For this review, take the finished solid that the model builds, in its own axes (mm). Face numbers are marked on the shaded views. A direction names the side the tool comes from. Round coordinates to 2 decimals unless told otherwise and drop trailing zeros. Loops run counter-clockwise (first coordinate to the right, second up) from the corner with the lowest first, then second, coordinate; pieces in that order, holes last. Notation, with made-up numbers: M -11.5,-25 L 14.5,-25 A18 ccw 14.5,-19 Z; hole C 44,75 d7. An arc over 180 degrees is marked long. One line per question, with ' | ' between items. Start each with the question number.
1) We need section D-D (x = 5.25). Give the boundary of the cut face in (y, z), and give its area (3 significant figures).
2) For probe 1 along Z at (x, y) = (-1.5, 46); probe 2 along Y at (x, z) = (4, -2), list the stretches that pass through material, from the lowest coordinate up. Write a range as from..to.
3) We need section B-B (x = 1). Give the boundary of the cut face in (y, z).
4) For pin 1 Ø3 at (x, y) = (2.5, 55) entering from -Z; pin 2 Ø2 at (x, y) = (1, 42.5) entering from +Z; pin 3 Ø6 at (y, z) = (49, 0) entering from +X, all flat-tipped, find the tip position at first contact; note any pin that passes through.
5) We need section A-A (z = -0.5). Give the boundary of the cut face in (x, y), and give its area (3 significant figures).
6) For the marked faces 1, 2, 3, 4 and 5, list the 3-axis set-ups (+Z, -Z, +X, -X, +Y, -Y) from which the entire face can be reached by the end or side of a thin tool; tool diameter is ignored.
7) We need section C-C (y = 16). Give the boundary of the cut face in (x, z), and give its area (3 significant figures).
Autodesk Inventor part; units mm, degrees
ref_plane "YZ Plane" through (0, 0, 0) normal (1, 0, 0) x (0, 1, 0)
ref_plane "XZ Plane" through (0, 0, 0) normal (0, 1, 0) x (-1, 0, 0)
ref_plane "XY Plane" through (0, 0, 0) normal (0, 0, 1) x (1, 0, 0)
sketch "Szkic1" plane through (0, 0, 0) normal (0, 1, 0) x (-1, 0, 0)
  line L0 (-6, 6) -> (6, 6)
  line L1 (6, 6) -> (6, -6)
  line L2 (6, -6) -> (-6, -6)
  line L3 (-6, -6) -> (-6, 6)
  line L4 (-6, 6) -> (6, -6) construction
  line L5 (6, 6) -> (-6, -6) construction
  line L6 (-3.5, 3.5) -> (3.5, 3.5)
  line L7 (3.5, 3.5) -> (3.5, -3.5)
  line L8 (3.5, -3.5) -> (-3.5, -3.5)
  line L9 (-3.5, -3.5) -> (-3.5, 3.5)
  line L10 (-3.5, 3.5) -> (3.5, -3.5) construction
  line L11 (3.5, 3.5) -> (-3.5, -3.5) construction
  point P0 (0, 0)
  dimension "d0" = 12
  dimension "d1" = 12
  dimension "d2" = 7
  dimension "d3" = 7
extrude "Wyciągnięcie proste1" add sketch "Szkic1" along normal blind 72 contours L6 L7 L8 L9
extrude "Wyciągnięcie proste2" add sketch "Szkic1" against normal blind 2 contours L0 L1 L2 L3 | L6 L7 L8 L9
fillet "Zaokrąglenie1" radius 1.5 8 edges at (6, -1, 6) (6, -1, -6) (-6, -1, 6) (-6, -1, -6) (0, -2, -6) (6, -2, 0) (0, -2, 6) (-6, -2, 0)
fillet "Zaokrąglenie2" radius 1 4 edges at (3.5, 72, 0) (0, 72, 3.5) (0, 72, -3.5) (-3.5, 72, 0)
properties part number "kołek"
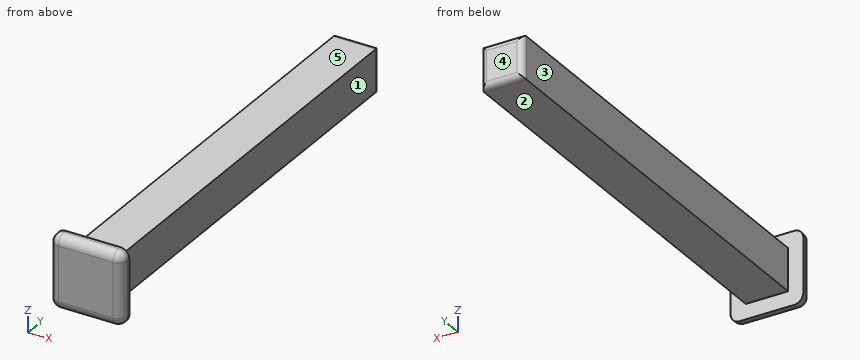
Answers below:
1) outline: M -1.8,-4.5 A1.3 ccw -0.5,-5.8 L 0,-5.8 L 0,5.8 L -0.5,5.8 A1.3 ccw -1.8,4.5 Z | area: 20.1 mm^2
2) probe 1: -3.5..3.5 | probe 2: -2..0
3) outline: M -2,-4.5 A1.5 ccw -0.5,-6 L 0,-6 L 0,-3.5 L 71,-3.5 A1 ccw 72,-2.5 L 72,2.5 A1 ccw 71,3.5 L 0,3.5 L 0,6 L -0.5,6 A1.5 ccw -2,4.5 Z
4) pin 1: z = -3.5 | pin 2: z = 3.5 | pin 3: x = 3.5
5) outline: M -6,-0.5 A1.5 ccw -4.5,-2 L 4.5,-2 A1.5 ccw 6,-0.5 L 6,0 L 3.5,0 L 3.5,71 A1 ccw 2.5,72 L -2.5,72 A1 ccw -3.5,71 L -3.5,0 L -6,0 Z | area: 527 mm^2
6) face 1: +Z, -Z, +X, +Y | face 2: -Z, +X, -X, +Y | face 3: +Z, -Z, -X, +Y | face 4: +Z, -Z, +X, -X, +Y | face 5: +Z, +X, -X, +Y
7) outline: M -3.5,-3.5 L 3.5,-3.5 L 3.5,3.5 L -3.5,3.5 Z | area: 49.0 mm^2
